```python
from build123d import *

# Parameters (mm, degrees)
F0_W     = 76.598722
F0_H     = 76.598718
F1_DEPTH = 152.4
F2_W     = 76.598719
F2_H     = 39.384769
F3_DEPTH = 50.8


with BuildPart() as f1:
    # F0 (on Front) → F1 (new body)
    with BuildSketch(Plane.XZ):
        with Locations((11.474302, -8.063022)):
            Rectangle(F0_W, F0_H)
    extrude(amount=-F1_DEPTH)

    # F2 (on Front) → F3 (join)
    with BuildSketch(Plane.XZ):
        with Locations((12.40465, -26.980116)):
            Rectangle(F2_W, F2_H)
    extrude(amount=F3_DEPTH)


solid = f1.part
```
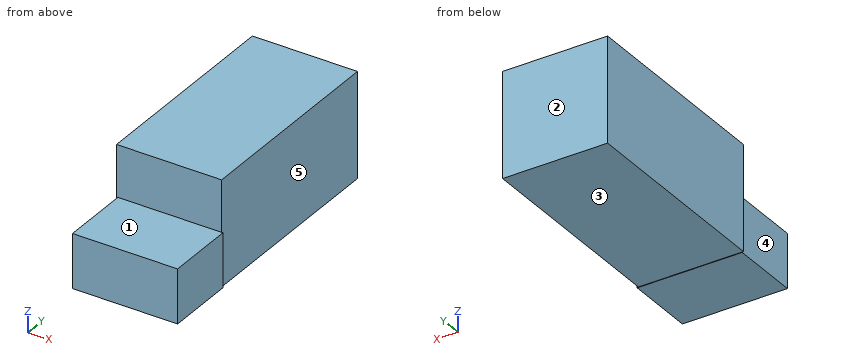
Here's how the part is built. I have some questions about the finished solid (model axes, mm). Face numbers are marked on the shaded views. A direction names the side the tool comes from. Give positions to 0.01 mm unless a question says otherwise; leave off trailing zeros. Write each loop counter-clockwise with the first axis right and the second up, starting at its lowest first coordinate (ties: lowest second). Pieces come first, ordered by that corner, then holes.
(1) Will these pins go through, and if not, where does the flat tip stop? pin 1 (1.5 mm diameter, centred on x = 13.5, y = 7.5, fed in from -Z); pin 2 (19.5 mm diameter, centred on y = -15, z = -32, fed in from -X); pin 3 (6 mm diameter, centred on x = -9, y = -9, fed in from +Z).
Output values:
pin 1: stops at z = -46.36
pin 2: stops at x = -25.89
pin 3: stops at z = -7.29
(2) Imagine slicing it at A-A, the plane x = 34. Write out the boundary of the cut face in (y, z), and give its area (3 significant figures).
Output values:
outline: (-50.8, -46.67) - (0, -46.67) - (0, -46.36) - (152.4, -46.36) - (152.4, 30.24) - (0, 30.24) - (0, -7.29) - (-50.8, -7.29) - close
area: 13,700 mm2
(3) On a 3-axis mill with a long thin cutter (end or side, diameter ignored), from which of +Z, -Z, +X, -X, +Y, -Y can I reach the whole of each face in a straight line? I mean the marked faces 1, 2, 3, 4 and 5. Say none if no direction works.
Output values:
face 1: +Z, +X, -X, -Y
face 2: +Z, -Z, +X, -X, +Y
face 3: -Z, +X, -X, +Y
face 4: +Z, -Z, -X, -Y
face 5: +Z, -Z, +X, +Y
(4) Imagine slicing it at C-C, the plane z = 14.5. Write out the boundary of the cut face in (x, y).
Output values:
outline: (-26.83, 0) - (49.77, 0) - (49.77, 152.4) - (-26.83, 152.4) - close
(5) If I drill on L1, parallel to X at y = 48, z = 16; L2, parallel to Z at x = 10.5, y = 51.5; L3, parallel to Z at x = 42, y = -19, over which ranges is the centre line in solid material (lowest first)?
Output values:
L1: x = -26.83 to 49.77
L2: z = -46.36 to 30.24
L3: z = -46.67 to -7.29
(6) Imagine slicing it at B-B, the plane y = 94. Write out the boundary of the cut face in (x, z), and give its area (3 significant figures).
Output values:
outline: (-26.83, -46.36) - (49.77, -46.36) - (49.77, 30.24) - (-26.83, 30.24) - close
area: 5,870 mm2
